Read the model definition and answer for the solid it produces. Units are mm, in the model's axes. Face numbers are marked on the shaded views. A direction names the side the tool comes from. Coordinates: 2 decimals unless noted, no trailing zeros. Write each loop counter-clockwise with the first axis right and the second up, starting at its lowest first coordinate (ties: lowest second). Pieces come first, ordered by that corner, then holes. Notation, with made-up numbers: (75.25, -12) -> (122.25, -12) arc R22 cw to (122.25, 4) -> close; hole circle Ø1 at (59, -37.75). An arc over 180 degrees is marked (long way). Use CSV: the item, a comma, the result in double quotes.
from build123d import *

# Parameters (mm, degrees)
BOSS_EXTRUDE1_DEPTH = 18
SKETCH2_R           = 1.5
CUT_EXTRUDE1_DEPTH  = 2
SKETCH3_R           = 0.8
CUT_EXTRUDE2_DEPTH  = 25.6018292
SKETCH4_R           = 0.8
CUT_EXTRUDE3_DEPTH  = 21.892582574


with BuildPart() as part:
    # Sketch1 → Boss-Extrude1 (new body)
    with BuildSketch(Plane(origin=(0, 0, 0), x_dir=(1, 0, 0), z_dir=(0, 1, 0))):
        with BuildLine():
            Line((0, 7.5), (7, 7.5))
            Line((7, 7.5), (7, 7))
            Line((7, 7), (0, 7))
            ThreePointArc((0, 7), (-7, 0), (0, -7))
            Line((0, -7), (7, -7))
            Line((7, -7), (7, -7.5))
            Line((7, -7.5), (0, -7.5))
            ThreePointArc((0, -7.5), (-7.5, 0), (0, 7.5))
        make_face()
    extrude(amount=BOSS_EXTRUDE1_DEPTH)

    # Sketch2 → Cut-Extrude1 (cut)
    with BuildSketch(Plane(origin=(0, 0, 7.5), x_dir=(-1, 0, 0), z_dir=(0, 0, -1))):
        with Locations(Location((-4, 14.5, 0), (0, 0, 180))):
            Circle(SKETCH2_R)
    extrude(amount=CUT_EXTRUDE1_DEPTH, mode=Mode.SUBTRACT)

    # Sketch3 → Cut-Extrude2 (cut, through all)
    with BuildSketch(Plane(origin=(0, 0, -7.5), x_dir=(-1, 0, 0), z_dir=(0, 0, -1))):
        with Locations((-5.5, 1.5)):
            Circle(SKETCH3_R)
        with Locations((-3, 1.5)):
            Circle(SKETCH3_R)
        with Locations(Location((-0.5, 1.5, 0), (0, 0, 51.317812547))):
            Circle(SKETCH3_R)
        with Locations((2, 1.5)):
            Circle(SKETCH3_R)
    extrude(amount=-CUT_EXTRUDE2_DEPTH, mode=Mode.SUBTRACT)

    # Sketch4 → Cut-Extrude3 (cut, through all)
    with BuildSketch(Plane(origin=(0, 0, 0), x_dir=(0, 0, -1), z_dir=(1, 0, 0))):
        with Locations((0, 1.5)):
            Circle(SKETCH4_R)
        with Locations((2.5, 1.5)):
            Circle(SKETCH4_R)
        with Locations((5, 1.5)):
            Circle(SKETCH4_R)
        with Locations((-2.5, 1.5)):
            Circle(SKETCH4_R)
        with Locations((-5, 1.5)):
            Circle(SKETCH4_R)
    extrude(amount=-CUT_EXTRUDE3_DEPTH, mode=Mode.SUBTRACT)


solid = part.part
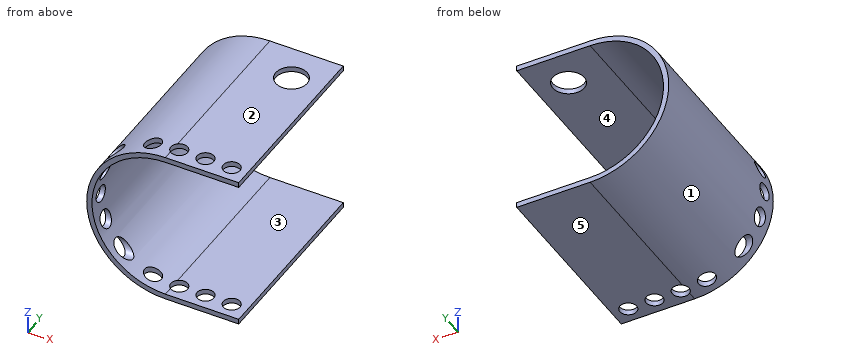
1. A cutting plane is placed at C-C (x = 3). Give the vertices of the cut face in (y, z).
Solutions:
outline,"(0, -7.5) -> (0.7, -7.5) -> (0.7, -7) -> (0, -7) -> close; (0, 7) -> (0.7, 7) -> (0.7, 7.5) -> (0, 7.5) -> close; (2.3, -7.5) -> (18, -7.5) -> (18, -7) -> (2.3, -7) -> close; (2.3, 7) -> (13.38, 7) -> (13.38, 7.5) -> (2.3, 7.5) -> close; (15.62, 7) -> (18, 7) -> (18, 7.5) -> (15.62, 7.5) -> close"
2. Each of these flat-tipped pins is pushed along its axis until it touches: pin 1 Ø2.5 at (y, z) = (1.5, 2.5) entering from +X; pin 2 Ø1 at (x, y) = (4, 14) entering from +Z; pin 3 Ø1.8 at (x, y) = (-2, 1.5) entering from -Z. Where does it stop, or does it pass through?
Solutions:
pin 1,"stops at x = -5.91"
pin 2,"stops at z = -7"
pin 3,"stops at z = -7.42"
3. A tool of negligible diameter and unlimited length cuts with its end or side. For the marked faces 4 and 5, from which of +Z, -Z, +X, -X, +Y, -Y can it reach the whole face along a straight path? Write none if from no direction.
Solutions:
face 4,"+X, +Y, -Y"
face 5,"-Z, +X, -X, +Y, -Y"
4. A cutting plane is placed at A-A (z = 0). Give the vertices of the cut face in (x, y), and give its area (3 significant figures).
Solutions:
outline,"(-7.5, 0) -> (-7, 0) -> (-7, 0.7) -> (-7.5, 0.7) -> close; (-7.5, 2.3) -> (-7, 2.3) -> (-7, 18) -> (-7.5, 18) -> close"
area,"8.20 mm^2"
5. For a pull along Z with two mould halves and no side action, classify the marked faces 1, 2 and 3 as pulls with the +Z half, pulls with the -Z half, needs draft (parallel to the pull), parting line crosses it, or undercut.
Solutions:
face 1,"parting line crosses it"
face 2,"pulls with the +Z half"
face 3,"undercut"
6. A cutting plane is placed at D-D (x = 0.75). Give the vertices of the cut face in (y, z), and give its area (3 significant figures).
Solutions:
outline,"(0, -7.5) -> (0.74, -7.5) -> (0.74, -7) -> (0, -7) -> close; (0, 7) -> (0.74, 7) -> (0.74, 7.5) -> (0, 7.5) -> close; (2.26, -7.5) -> (18, -7.5) -> (18, -7) -> (2.26, -7) -> close; (2.26, 7) -> (18, 7) -> (18, 7.5) -> (2.26, 7.5) -> close"
area,"16.5 mm^2"
7. A cutting plane is placed at B-B (y = 8.75). Give the vertices of the cut face in (x, z), and give its area (3 significant figures).
Solutions:
outline,"(0, -7.5) -> (7, -7.5) -> (7, -7) -> (0, -7) arc R7 cw to (0, 7) -> (7, 7) -> (7, 7.5) -> (0, 7.5) arc R7.5 ccw to start"
area,"18.4 mm^2"
8. Find the intervals of material crossed by line 1 along Z through (x, y) = (2, 8.25); line 2 along Y through (x, z) = (3, -7.2); line 3 along Y through (x, z) = (4, 7.25), in increasing order.
Solutions:
line 1,"z = -7.5 to -7, 7 to 7.5"
line 2,"y = 0 to 0.7, 2.3 to 18"
line 3,"y = 0 to 13, 16 to 18"
